Model file for the job. Use its own axes, mm. A direction names the side the tool comes from. Coordinates: 2 decimals unless noted, no trailing zeros. Loops run counter-clockwise (first coordinate to the right, second up) from the corner with the lowest first, then second, coordinate; pieces in that order, holes last. Notation, with made-up numbers: (2, -16.5) - (39, -16.5) arc R17 cw to (39, 0.5) - close; hole circle Ø3 at (24, -35). An arc over 180 degrees is marked (long way). Write each question's results on one line, items separated by ' | '. Start each with the question number.
```python
from build123d import *

# Parameters (mm, degrees)
SKETCH_1_W          = 200
SKETCH_1_H          = 52
EXTRUDE_1_DEPTH     = 18
CUT_EXTRUDE_1_DEPTH = 203.484567313
SKETCH_3_W          = 196
SKETCH_3_H          = 12
CUT_EXTRUDE_2_DEPTH = 16
HOLE_WIZARD_M5_1_D  = 5.5
SKETCH_6_W          = 41
SKETCH_6_H          = 16
EXTRUDE_2_DEPTH     = 20


with BuildPart() as part:
    # 草图1 → 凸台-拉伸1 (new body)
    with BuildSketch(Plane.XY):
        Rectangle(SKETCH_1_W, SKETCH_1_H)
    extrude(amount=EXTRUDE_1_DEPTH)

    # 草图2 → 切除-拉伸1 (cut, through all)
    with BuildSketch(Plane.ZY.offset(100)):
        Polygon((18, 14), (6, 26), (18, 26), align=None)
    extrude(amount=-CUT_EXTRUDE_1_DEPTH, mode=Mode.SUBTRACT)

    # 草图3 → 切除-拉伸2 (cut)
    with BuildSketch(Plane.XY.offset(18)):
        with Locations((0, 20)):
            Rectangle(SKETCH_3_W, SKETCH_3_H)
    extrude(amount=-CUT_EXTRUDE_2_DEPTH, mode=Mode.SUBTRACT)

    # M5 间隙孔1 (through all)
    with Locations(Plane.XY.offset(2)):
        with Locations((-50, 20), (50, 20), (70, 20), (-70, 20)):
            Hole(HOLE_WIZARD_M5_1_D / 2)

    # 草图6 → 凸台-拉伸2 (add)
    with BuildSketch(Plane.XY.offset(2)):
        with Locations((0, 22)):
            Rectangle(SKETCH_6_W, SKETCH_6_H)
    extrude(amount=EXTRUDE_2_DEPTH)


solid = part.part
```
Q1. Pin check, flat tips, straight feed: pin 1 (13 mm diameter, centred on x = -45, z = 13, fed in from +Y); pin 2 (3.5 mm diameter, centred on x = 47, y = 18, fed in from +Z); pin 3 (6.5 mm diameter, centred on x = 28.5, z = 3, fed in from +Y); pin 4 (3.5 mm diameter, centred on x = 70, y = 20, fed in from +Z). Stop position of each tip, or through.
Q2. Mould opens along X. For faces 4 (the flat face through (0, 14, 20)), 5 (the flat face through (100, 0, 9)), 6 (the cylindrical face through (52.747, 20.121, 0.986)) say: +X half, -X half, draft (parallel to the pull), parting line (faces both ways), or undercut.
Q3. Cut at C-C (z = 15). List the corners of the cut face in (x, y), and give its area (3 significant figures).
Q4. Which spindle directions (+Z, -Z, +X, -X, +Y, -Y) get a long thin tool onto all of the face, cutting with end or side? Do faces 1 (the flat face through (-99, 20, 12)), 2 (the flat face through (-20.5, 22, 12)), 3 (the flat face through (0, 28, 2)). Say none if no direction does.
Q5. Drill centre lines: L1, parallel to X at y = 20.5, z = 4.25; L2, parallel to Y at x = 50, z = 0.5; L3, parallel to Z at x = 83, y = 1. Where is each one in solid material? Low to high. Write a range as from..to.
Q6. Cut at B-B (y = 20). List the corners of the cut face in (x, z).
Q7. Cut at D-D (x = -54.5). List the corners of the cut face in (y, z), and give its area (3 significant figures).
Q8. Cut at A-A (x = 70). List the corners of the cut face in (y, z), and give its area (3 significant figures).
Check result:
1) pin 1: y = 14 | pin 2: z = 2 | pin 3: y = 26 | pin 4: through
2) face 4: draft | face 5: +X half | face 6: undercut
3) outline: (-100, -26) - (100, -26) - (100, 17) - (98, 17) - (98, 14) - (20.5, 14) - (20.5, 30) - (-20.5, 30) - (-20.5, 14) - (-98, 14) - (-98, 17) - (-100, 17) - close | area: 8,670 mm²
4) face 1: +Z, -X, +Y | face 2: +Z, +Y | face 3: -Z, +X, -X, +Y
5) L1: -100..-98, -20.5..20.5, 98..100 | L2: -26..17.25, 22.75..26 | L3: 0..18
6) outline: (-100, 0) - (-72.75, 0) - (-72.75, 2) - (-98, 2) - (-98, 12) - (-100, 12) - close; (-67.25, 0) - (-52.75, 0) - (-52.75, 2) - (-67.25, 2) - close; (-47.25, 0) - (47.25, 0) - (47.25, 2) - (20.5, 2) - (20.5, 22) - (-20.5, 22) - (-20.5, 2) - (-47.25, 2) - close; (52.75, 0) - (67.25, 0) - (67.25, 2) - (52.75, 2) - close; (72.75, 0) - (100, 0) - (100, 12) - (98, 12) - (98, 2) - (72.75, 2) - close
7) outline: (-26, 0) - (26, 0) - (26, 2) - (14, 2) - (14, 18) - (-26, 18) - close | area: 744 mm²
8) outline: (-26, 0) - (17.25, 0) - (17.25, 2) - (14, 2) - (14, 18) - (-26, 18) - close; (22.75, 0) - (26, 0) - (26, 2) - (22.75, 2) - close | area: 733 mm²
